Here's how the part is built. I have some questions about the finished solid (model axes, mm). A direction names the side the tool comes from. Round coordinates to 2 decimals unless told otherwise and drop trailing zeros. Order: outer loops, then holes, each group sorted by start corner. A loop starts at its lowest first (then second) coordinate and runs counter-clockwise, first axis right, second up. Notation, with made-up numbers: (-15.75, 59.5) - (7.25, 59.5) arc R14 ccw to (7.25, 86.5) - close; hole circle Ø6 at (67, 58.5). An arc over 180 degrees is marked (long way). One line per item, written item: value.
from build123d import *

# Parameters (mm, degrees)
SKETCH1_W           = 90
SKETCH1_H           = 55
BOSS_EXTRUDE1_DEPTH = 55
SHELL1_T            = -2
SKETCH2_W           = 4
SKETCH2_H           = 55
BOSS_EXTRUDE2_DEPTH = 88
SKETCH3_W           = 4
SKETCH3_H           = 49
CUT_EXTRUDE1_DEPTH  = 60
SKETCH4_W           = 1.2
SKETCH4_H           = 52
CUT_EXTRUDE2_DEPTH  = 61.5
CUT_EXTRUDE3_START  = -10
SKETCH5_W           = 13
SKETCH5_H           = 19.5
CUT_EXTRUDE3_DEPTH  = 46
SKETCH7_R           = 5
BOSS_EXTRUDE3_DEPTH = 5
SKETCH8_R           = 1.4
CUT_EXTRUDE4_DEPTH  = 5
BOSS_EXTRUDE4_REACH = 90
SKETCH9_W           = 4
SKETCH9_H           = 51


with BuildPart() as part:
    # Sketch1 → Boss-Extrude1 (new body)
    with BuildSketch(Plane.XY):
        Rectangle(SKETCH1_W, SKETCH1_H)
    extrude(amount=BOSS_EXTRUDE1_DEPTH)

    # Shell1
    shell1_openings = [part.faces().sort_by_distance(p)[0] for p in [
        (0, 0, 55),
    ]]
    offset(amount=SHELL1_T, openings=shell1_openings, kind=Kind.INTERSECTION)

    # Sketch2 → Boss-Extrude2 (add)
    with BuildSketch(Plane(origin=(45, 0, 0), x_dir=(0, 0, -1), z_dir=(1, 0, 0))):
        with Locations((-53, 0)):
            Rectangle(SKETCH2_W, SKETCH2_H)
    extrude(amount=-BOSS_EXTRUDE2_DEPTH)

    # Sketch3 → Cut-Extrude1 (cut)
    with BuildSketch(Plane(origin=(45, 0, 0), x_dir=(0, 0, -1), z_dir=(1, 0, 0))):
        with Locations((-53, 0)):
            Rectangle(SKETCH3_W, SKETCH3_H)
    extrude(amount=-CUT_EXTRUDE1_DEPTH, mode=Mode.SUBTRACT)

    # Sketch4 → Cut-Extrude2 (cut)
    with BuildSketch(Plane(origin=(45, 0, 0), x_dir=(0, 0, -1), z_dir=(1, 0, 0))):
        with Locations((-53, 0)):
            Rectangle(SKETCH4_W, SKETCH4_H)
    extrude(amount=-CUT_EXTRUDE2_DEPTH, mode=Mode.SUBTRACT)

    # Sketch5 → Cut-Extrude3 (cut, through all)
    with BuildSketch(Plane.XY.offset(55).offset(CUT_EXTRUDE3_START)):
        with Locations((-32.5, -0.25)):
            Rectangle(SKETCH5_W, SKETCH5_H)
    extrude(amount=-CUT_EXTRUDE3_DEPTH, mode=Mode.SUBTRACT)

    # Sketch7 → Boss-Extrude3 (add)
    with BuildSketch(Plane.XY.offset(2)):
        with Locations((3, 19.5)):
            Circle(SKETCH7_R)
        with Locations((-13, -9)):
            Circle(SKETCH7_R)
        with Locations((13, 17.5)):
            Circle(SKETCH7_R)
        with Locations((37, -6.5)):
            Circle(SKETCH7_R)
    extrude(amount=BOSS_EXTRUDE3_DEPTH)

    # Sketch8 → Cut-Extrude4 (cut)
    with BuildSketch(Plane.XY.offset(7)):
        with Locations((13, 17.5)):
            Circle(SKETCH8_R)
        with Locations((-13, -9)):
            Circle(SKETCH8_R)
        with Locations((37, -6.5)):
            Circle(SKETCH8_R)
        with Locations((3, 19.5)):
            Circle(SKETCH8_R)
    extrude(amount=-CUT_EXTRUDE4_DEPTH, mode=Mode.SUBTRACT)

    # Sketch9 → Boss-Extrude4 (add, up to next)
    with BuildSketch(Plane(origin=(-43, 0, 0), x_dir=(0, 0, -1), z_dir=(1, 0, 0)), mode=Mode.PRIVATE) as boss_extrude4_sk1:
        with Locations((-35.5, 0)):
            Rectangle(SKETCH9_W, SKETCH9_H)
    boss_extrude4_tool1 = extrude(boss_extrude4_sk1.sketch, amount=BOSS_EXTRUDE4_REACH, mode=Mode.PRIVATE) - part.part
    add(boss_extrude4_tool1.solids().sort_by_distance((-43, 0, 35.5))[0])


solid = part.part
Q1. If we section it at D-D, the plane x = -32: Please give me the cut outline in (y, z), then the cut area to 3 significant figures.
Results list:
outline: (-27.5, 0) - (-10, 0) - (-10, 2) - (-25.5, 2) - (-25.5, 33.5) - (25.5, 33.5) - (25.5, 2) - (9.5, 2) - (9.5, 0) - (27.5, 0) - (27.5, 55) - (-27.5, 55) - close; hole (-25.5, 37.5) - (25.5, 37.5) - (25.5, 51) - (-25.5, 51) - close
area: 691 mm²
Q2. Will these pins go through, and if not, where does the flat tip stop? pin 1 (1 mm diameter, centred on x = -31.5, y = -0.5, fed in from -Z); pin 2 (1 mm diameter, centred on x = 43.5, y = 5, fed in from +Z); pin 3 (3 mm diameter, centred on x = -11, y = -6.5, fed in from +Z).
Results list:
pin 1: z = 33.5
pin 2: z = 51
pin 3: z = 37.5
Q3. Which directions (+Z, -Z, +X, -X, +Y, -Y) give clear straight access to the entire face, cutting with the end or side of a thin tool? Please do faces 1 (the flat face through (-33, -10, 1)), 2 (the flat face through (-15.2, -0.1, 53.6)), 3 (the cylindrical face through (1.92, 14.62, 4.46)), 4 (the flat face through (-21, 6, 55)).
Results list:
face 1: -Z
face 2: +X
face 3: none
face 4: +Z, +X, -X, +Y, -Y
Q4. If I drill on line 1 along Y through (x, z) = (13, 4); line 2 along Y through (x, z) = (4, 41); line 3 along X through (y, z) = (0.5, 5), over which ranges is the centre line in solid material (lowest first)?
Results list:
line 1: -27.5 to -25.5, 12.5 to 16.1, 18.9 to 22.5, 25.5 to 27.5
line 2: -27.5 to -25.5, 25.5 to 27.5
line 3: -45 to -43, 43 to 45
Q5. We'd pull the mould along Y, two halves only. Please class faces 5 (the flat face through (45, 0, 27)), 6 (the flat face through (-1, 0, 33.5)): released by +Y, released by -Y, zero draft, split by the parting line, or undercut.
Results list:
face 5: zero draft
face 6: undercut
Q6. If we section it at C-C, the plane z = 25.5: Please give me the cut outline in (x, y), then the cut area to 3 significant figures.
Results list:
outline: (-45, -27.5) - (45, -27.5) - (45, 27.5) - (-45, 27.5) - close; hole (-43, -25.5) - (43, -25.5) - (43, 25.5) - (-43, 25.5) - close
area: 564 mm²
Q7. If we section it at B-B, the plane y = -18: Please give me the cut outline in (x, z).
Results list:
outline: (-45, 0) - (45, 0) - (45, 51) - (43, 51) - (43, 37.5) - (-43, 37.5) - (-43, 51) - (-15, 51) - (-15, 52.4) - (-16.5, 52.4) - (-16.5, 53.6) - (-15, 53.6) - (-15, 55) - (-45, 55) - close; hole (-43, 2) - (43, 2) - (43, 33.5) - (-43, 33.5) - close
Q8. If we section it at A-A, the plane x = 25: Please give me the cut outline in (y, z), then the cut area to 3 significant figures.
Results list:
outline: (-27.5, 0) - (27.5, 0) - (27.5, 55) - (24.5, 55) - (24.5, 53.6) - (26, 53.6) - (26, 52.4) - (24.5, 52.4) - (24.5, 51) - (25.5, 51) - (25.5, 37.5) - (-25.5, 37.5) - (-25.5, 51) - (-24.5, 51) - (-24.5, 52.4) - (-26, 52.4) - (-26, 53.6) - (-24.5, 53.6) - (-24.5, 55) - (-27.5, 55) - close; hole (-25.5, 2) - (25.5, 2) - (25.5, 33.5) - (-25.5, 33.5) - close
area: 530 mm²
